Design review of the part built by this model. Coordinates are the model's own, in mm. A direction names the side the tool comes from. Coordinates: 2 decimals unless noted, no trailing zeros. Write each loop counter-clockwise with the first axis right and the second up, starting at its lowest first coordinate (ties: lowest second). Pieces come first, ordered by that corner, then holes. Notation, with made-up numbers: M -18,20 L 30,20 A37 ccw 30,57 Z; hole C 31.5,-27.75 d3. An arc over 180 degrees is marked long. Write each question's results on one line, items separated by ' | '. Start each with the question number.
```python
from build123d import *

# Parameters (mm, degrees)
BOSS_EXTRUDE1_DEPTH = 5
CUT_EXTRUDE2_DEPTH  = 6


with BuildPart() as part:
    # Sketch1 → Boss-Extrude1 (new body)
    with BuildSketch(Plane.XY):
        Polygon((-13.5, 0), (13.5, 0), (13.5, 24), (18.5, 24), (18.5, 49), (13.5, 49), (13.5, 64), (-13.5, 64), (-13.5, 49), (-18.5, 49), (-18.5, 24), (-13.5, 24), align=None)
    extrude(amount=BOSS_EXTRUDE1_DEPTH)

    # Sketch2 → Cut-Extrude2 (cut, through all)
    with BuildSketch(Plane.XY.offset(5)):
        Polygon((-13.5, 56.5), (-13.5, 57.7), (-9.5, 57.7), (-9.5, 59.25), (-7.7, 59.25), (-7.7, 57.654169795), (-5.7, 57.654169795), (-5.7, 55.345830205), (-7.7, 55.345830205), (-7.7, 53.75), (-9.5, 53.75), (-9.5, 55.3), (-13.5, 55.3), align=None)
        Polygon((13.5, 56.5), (13.5, 55.3), (9.5, 55.3), (9.5, 53.75), (7.7, 53.75), (7.7, 55.345830205), (5.7, 55.345830205), (5.7, 57.654169795), (7.7, 57.654169795), (7.7, 59.25), (9.5, 59.25), (9.5, 57.7), (13.5, 57.7), align=None)
        Polygon((-13.5, 10.8), (-13.5, 13.2), (-9.5, 13.2), (-9.5, 14.75), (-7.7, 14.75), (-7.7, 13.2), (-5.7, 13.2), (-5.7, 10.8), (-7.7, 10.8), (-7.7, 9.25), (-9.5, 9.25), (-9.5, 10.8), align=None)
        Polygon((13.5, 10.8), (9.5, 10.8), (9.5, 9.25), (7.7, 9.25), (7.7, 10.8), (5.7, 10.8), (5.7, 13.2), (7.7, 13.2), (7.7, 14.75), (9.5, 14.75), (9.5, 13.2), (13.5, 13.2), align=None)
    extrude(amount=-CUT_EXTRUDE2_DEPTH, mode=Mode.SUBTRACT)


solid = part.part
```
Item 1: Draft analysis for pull direction Y (two halves, no side actions). For faces 6 (the flat face through (0, 64, 2)), 7 (the flat face through (11, 13.2, 3)), 8 (the flat face through (-13.5, 19, 2)), state which applies: released by +Y, released by -Y, zero draft, split by the parting line, or undercut.
Item 2: For faces 1 (the flat face through (-9, 9.25, 3)), 2 (the flat face through (-11, 10.8, 3)), 3 (the flat face through (7, 13.2, 3)), 4 (the flat face through (18.5, 36, 2)), 5 (the flat face through (13.5, 52, 2)), list the 3-axis set-ups (+Z, -Z, +X, -X, +Y, -Y) from which the entire face can be reached by the end or side of a thin tool; tool diameter is ignored.
Item 3: We need section A-A on x = -12.5. State the section outline as (y, z) points, then the cut area to 3 significant figures.
Item 4: We need section B-B on x = 6.5. State the section outline as (y, z) points.
Item 5: Insertion check: pin 1 Ø1.5 at (y, z) = (17, 1.5) entering from -X; pin 2 Ø12 at (x, y) = (4, 55.5) entering from -Z; pin 3 Ø1.2 at (y, z) = (12.5, 2) entering from -X; pin 4 Ø0.7 at (y, z) = (56.5, 2) entering from +X. Each pin has a flat end and moves straight along its axis. Give the tip position at first contact, or say it passes through.
Item 6: Wall thickness on L1, parallel to X at y = 58.5, z = 0.9; L2, parallel to Y at x = 11.5, z = 1.9; L3, parallel to Y at x = 8, z = 2.05: over which ranges is each line inside the solid? List them lowest first.
Item 7: We need section C-C on y = 19.5. State the section outline as (x, z) points, then the cut area to 3 significant figures.
Item 8: We need section D-D on y = 56. State the section outline as (x, z) points.
Answer:
1) face 6: released by +Y | face 7: undercut | face 8: zero draft
2) face 1: +Z, -Z | face 2: +Z, -Z, -X | face 3: +Z, -Z, +X | face 4: +Z, -Z, +X, +Y, -Y | face 5: +Z, -Z, +X, +Y
3) outline: M 0,0 L 10.8,0 L 10.8,5 L 0,5 Z; M 13.2,0 L 55.3,0 L 55.3,5 L 13.2,5 Z; M 57.7,0 L 64,0 L 64,5 L 57.7,5 Z | area: 296 mm^2
4) outline: M 0,0 L 10.8,0 L 10.8,5 L 0,5 Z; M 13.2,0 L 55.35,0 L 55.35,5 L 13.2,5 Z; M 57.65,0 L 64,0 L 64,5 L 57.65,5 Z
5) pin 1: stops at x = -13.5 | pin 2: stops at z = 0 | pin 3: stops at x = -5.7 | pin 4: stops at x = 5.7
6) L1: x = -13.5 to -9.5, -7.7 to 7.7, 9.5 to 13.5 | L2: y = 0 to 10.8, 13.2 to 55.3, 57.7 to 64 | L3: y = 0 to 9.25, 14.75 to 53.75, 59.25 to 64
7) outline: M -13.5,0 L 13.5,0 L 13.5,5 L -13.5,5 Z | area: 135 mm^2
8) outline: M -5.7,0 L 5.7,0 L 5.7,5 L -5.7,5 Z
